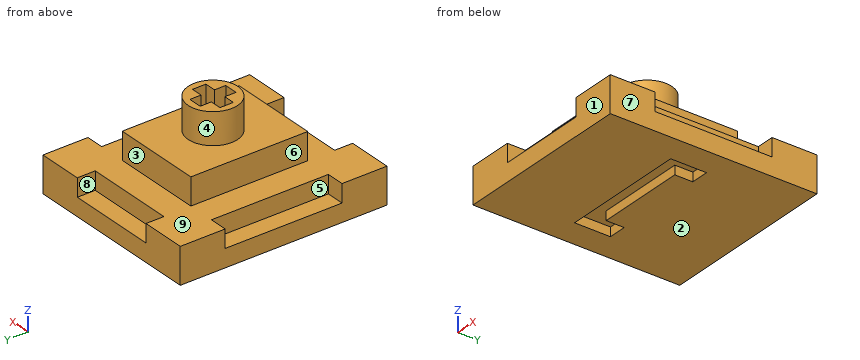
Autodesk Fusion 360 part; units mm, degrees
sketch "スケッチ1" plane through (0, 0, 0) normal (0, 0, 1) x (1, 0, 0)
  line L0 (0, 0) -> (20, 0)
  line L1 (20, 0) -> (20, 23)
  line L2 (20, 23) -> (0, 23)
  line L3 (0, 23) -> (0, 0)
  dimension "d1" = 20
  dimension "d2" = 23
extrude "押し出し1" add sketch "スケッチ1" along normal blind 2
sketch "スケッチ2" plane through (0, 0, 2) normal (0, 0, 1) x (-1, 0, 0)
  line L0 (0, -23) -> (0, 0)
  line L1 (0, 0) -> (-20, 0)
  line L2 (-20, 0) -> (-20, -23)
  line L3 (-20, -23) -> (0, -23)
  line L4 (0, -23) -> (-5, -23)
  line L5 (-5, -23) -> (-5, -18)
  line L6 (-5, -18) -> (0, -18)
  line L7 (0, -18) -> (0, -23)
  line L8 (-20, -23) -> (-15, -23)
  line L9 (-15, -23) -> (-15, -18)
  line L10 (-15, -18) -> (-20, -18)
  line L11 (-20, -18) -> (-20, -23)
  line L12 (0, 0) -> (-5, 0)
  line L13 (-5, 0) -> (-5, -5)
  line L14 (-5, -5) -> (0, -5)
  line L15 (0, -5) -> (0, 0)
  line L16 (-20, 0) -> (-15, 0)
  line L17 (-15, 0) -> (-15, -5)
  line L18 (-15, -5) -> (-20, -5)
  line L19 (-20, -5) -> (-20, 0)
  line L20 (-2, -21) -> (-18, -21)
  line L21 (-18, -21) -> (-18, -2)
  line L22 (-18, -2) -> (-2, -2)
  line L23 (-2, -2) -> (-2, -21)
  dimension "d5" = 5
  dimension "d6" = 5
  dimension "d7" = 5
  dimension "d8" = 5
  dimension "d9" = 5
  dimension "d10" = 5
  dimension "d11" = 5
  dimension "d12" = 5
extrude "押し出し2" add sketch "スケッチ2" along normal blind 2 contours L0 L3 L4 L5 L6 L7 L20 L23 | L0 L1 L12 L13 L14 L15 L22 L23 | L5 L6 L20 L23 | L5 L6 L9 L10 L13 L14 L17 L18 L20 L21 L22 L23 | L2 L3 L8 L9 L10 L11 L20 L21 | L13 L14 L22 L23 | L9 L10 L20 L21 | L1 L2 L16 L17 L18 L19 L21 L22 | L17 L18 L21 L22
sketch "スケッチ3" plane through (0, 0, 4) normal (0, 0, 1) x (-1, 0, 0)
  line L0 (-18, -18) -> (-20, -18)
  line L1 (-20, -18) -> (-20, -23)
  line L2 (-20, -23) -> (-15, -23)
  line L3 (-15, -23) -> (-15, -21)
  line L4 (-15, -21) -> (-5, -21)
  line L5 (-5, -21) -> (-5, -23)
  line L6 (-5, -23) -> (0, -23)
  line L7 (0, -23) -> (0, -18)
  line L8 (0, -18) -> (-2, -18)
  line L9 (-2, -18) -> (-2, -5)
  line L10 (-2, -5) -> (0, -5)
  line L11 (0, -5) -> (0, 0)
  line L12 (0, 0) -> (-5, 0)
  line L13 (-5, 0) -> (-5, -2)
  line L14 (-5, -2) -> (-15, -2)
  line L15 (-15, -2) -> (-15, 0)
  line L16 (-15, 0) -> (-20, 0)
  line L17 (-20, 0) -> (-20, -5)
  line L18 (-20, -5) -> (-18, -5)
  line L19 (-18, -5) -> (-18, -18)
  line L20 (-5, -18) -> (-15, -18)
  line L21 (-15, -18) -> (-15, -5)
  line L22 (-15, -5) -> (-5, -5)
  line L23 (-5, -5) -> (-5, -18)
extrude "押し出し3" add sketch "スケッチ3" along normal blind 3 contours L20 L21 L22 L23
sketch "スケッチ4" plane through (0, 0, 7) normal (0, 0, 1) x (-1, 0, 0)
  line L0 (-5, -5) -> (-15, -5)
  line L1 (-15, -5) -> (-15, -18)
  line L2 (-15, -18) -> (-5, -18)
  line L3 (-5, -18) -> (-5, -5)
  line L4 (-9.55, -13.5) -> (-11.05, -13.5)
  line L5 (-11.05, -13.5) -> (-11.05, -9.5)
  line L6 (-11.05, -9.5) -> (-9.55, -9.5)
  line L7 (-9.55, -9.5) -> (-9.55, -13.5)
  line L8 (-8.3, -12.25) -> (-12.3, -12.25)
  line L9 (-12.3, -12.25) -> (-12.3, -10.75)
  line L10 (-12.3, -10.75) -> (-8.3, -10.75)
  line L11 (-8.3, -10.75) -> (-8.3, -12.25)
  circle A0 centre (-10.3, -11.5) radius 2.75
  dimension "d17" = 13
  dimension "d18" = 1.5
  dimension "d19" = 4
  dimension "d20" = 4
  dimension "d21" = 1.5
  dimension "d22" = 5.5
extrude "押し出し4" add sketch "スケッチ4" along normal blind 3.5 contours A0
sketch "スケッチ7" plane through (0, 0, 0) normal (0, 0, -1) x (1, 0, 0)
  line L0 (0, 0) -> (0, -23)
  line L1 (0, -23) -> (20, -23)
  line L2 (20, -23) -> (20, 0)
  line L3 (20, 0) -> (0, 0)
  line L4 (17, -9) -> (17, -13)
  line L5 (15, -13) -> (15, -9)
  line L6 (15, -9) -> (17, -9)
  line L7 (17, -13) -> (15, -13)
  line L8 (5, -9) -> (15, -9)
  line L9 (15, -11) -> (5, -11)
  line L10 (5, -11) -> (5, -9)
  line L11 (15, -9) -> (15, -11)
  line L12 (5, -13) -> (3, -13)
  line L13 (3, -13) -> (3, -9)
  line L14 (3, -9) -> (5, -9)
  line L15 (5, -9) -> (5, -13)
extrude "押し出し7" cut sketch "スケッチ7" against normal blind 1 contours L4 L5 L6 L7 L11 | L5 L8 L9 L10 L11 L15 | L10 L12 L13 L14 L15
Verification items for the finished model (mm, model axes). Face numbers are marked on the shaded views. A direction names the side the tool comes from. Give positions to 0.01 mm unless a question says otherwise; leave off trailing zeros. Write each loop counter-clockwise with the first axis right and the second up, starting at its lowest first coordinate (ties: lowest second). Pieces come first, ordered by that corner, then holes.
(1) Cross-section at A-A (y = 16). Enter the section's corners in (x, z), plus the area to 3 significant figures.
(2) Mould release check, pull along X, two halves, no side actions. Record for the marked faces 6, 7, 8 and 9: +X half, -X half, draft (parallel to the pull), parting line (faces both ways), or undercut.
(3) Access from +Z, -Z, +X, -X, +Y, -Y to the whole of each face (thin tool, end or side, straight path). Record for the marked faces 1, 2, 3, 4 and 5.
(4) Cross-section at D-D (x = 16.5). Enter the section's corners in (y, z).
(5) Material ranges on line 1 (Z direction, x = 6, y = 18.5); line 2 (Y direction, x = 11.25, z = 6.25); line 3 (X direction, y = 14.25, z = 5.75), recorded low to high.
(6) Cross-section at C-C (x = 6.5). Enter the section's corners in (y, z), plus the area to 3 significant figures.
(7) Cross-section at B-B (z = 9.5). Enter the section's corners in (x, y), plus the area to 3 significant figures.
(8) Gauge pin test, flat ends, axial feed: pin 1 (0.6 mm diameter, centred on x = 1, y = 13.5, fed in from +Z); pin 2 (6 mm diameter, centred on y = 17, z = 8.5, fed in from -X); pin 3 (1 mm diameter, centred on x = 11.5, z = 3, fed in from -Y). Record the tip position at first contact, or that the pin passes through.
Worked out:
1. outline: (0, 0) - (20, 0) - (20, 2) - (18, 2) - (18, 4) - (15, 4) - (15, 7) - (5, 7) - (5, 4) - (2, 4) - (2, 2) - (0, 2) - close
1. area: 102 mm2
2. face 6: -X half
2. face 7: +X half
2. face 8: undercut
2. face 9: draft
3. face 1: +Z, -Z, +X, -X, -Y
3. face 2: -Z, +X, -X, +Y, -Y
3. face 3: +Z, +X, -X, +Y
3. face 4: +Z
3. face 5: +Z, -X
4. outline: (0, 0) - (9, 0) - (9, 1) - (13, 1) - (13, 0) - (23, 0) - (23, 4) - (0, 4) - close
5. line 1: z = 0 to 4
5. line 2: y = 5 to 18
5. line 3: x = 5 to 15
6. outline: (0, 0) - (9, 0) - (9, 1) - (11, 1) - (11, 0) - (23, 0) - (23, 2) - (21, 2) - (21, 4) - (18, 4) - (18, 7) - (5, 7) - (5, 4) - (2, 4) - (2, 2) - (0, 2) - close
6. area: 121 mm2
7. outline: circle Ø5.5 at (10.3, 11.5); hole (8.3, 10.75) - (9.55, 10.75) - (9.55, 9.5) - (11.05, 9.5) - (11.05, 10.75) - (12.3, 10.75) - (12.3, 12.25) - (11.05, 12.25) - (11.05, 13.5) - (9.55, 13.5) - (9.55, 12.25) - (8.3, 12.25) - close
7. area: 14.0 mm2
8. pin 1: stops at z = 2
8. pin 2: stops at x = 5
8. pin 3: stops at y = 2
